```python
from build123d import *

# Parameters (mm, degrees)
SKETCH1_W           = 30
SKETCH1_H           = 30
BOSS_EXTRUDE1_DEPTH = 1.6
SKETCH2_R           = 0.6
CUT_EXTRUDE1_DEPTH  = 1.6
CIRPATTERN1_COUNT   = 2
CIRPATTERN1_ANGLE   = 90
SKETCH4_R           = 0.6
BOSS_EXTRUDE2_DEPTH = 4


with BuildPart() as part:
    # Sketch1 → Boss-Extrude1 (new body)
    with BuildSketch(Plane(origin=(0, 0, 0), x_dir=(1, 0, 0), z_dir=(0, 1, 0))):
        with Locations((15, 15)):
            Rectangle(SKETCH1_W, SKETCH1_H)
    extrude(amount=BOSS_EXTRUDE1_DEPTH)

    # Sketch2 → Cut-Extrude1 (cut)
    with BuildSketch(Plane(origin=(0, 1.6, 0), x_dir=(1, 0, 0), z_dir=(0, 1, 0))):
        with Locations((20.5, 5)):
            Circle(SKETCH2_R)
        with Locations((9.5, 5)):
            Circle(SKETCH2_R)
        with Locations((20.5, 25)):
            Circle(SKETCH2_R)
        with Locations((9.5, 25)):
            Circle(SKETCH2_R)
    cut_extrude1 = extrude(amount=-CUT_EXTRUDE1_DEPTH, mode=Mode.SUBTRACT)

    # CirPattern1: Cut-Extrude1 ×2 about axis
    cirpattern1_axis = Axis((15, 0, -15), (0, 1, 0))
    for i in range(1, CIRPATTERN1_COUNT):
        add(cut_extrude1.rotate(cirpattern1_axis, i * CIRPATTERN1_ANGLE / (CIRPATTERN1_COUNT - 1)), mode=Mode.SUBTRACT)

    # Sketch4 → Boss-Extrude2 (add)
    with BuildSketch(Plane(origin=(0, 1.6, 0), x_dir=(1, 0, 0), z_dir=(0, 1, 0))):
        with Locations((15, 15)):
            Circle(SKETCH4_R)
    extrude(amount=BOSS_EXTRUDE2_DEPTH)


solid = part.part
```
Input: part model. Units: mm. Frame: model coordinates. Round coordinates to 2 decimals unless told otherwise and drop trailing zeros. Loops run counter-clockwise (first coordinate to the right, second up) from the corner with the lowest first, then second, coordinate; pieces in that order, holes last. Notation, with made-up numbers: (4.25, -40) -> (61.25, -40) arc R25 ccw to (61.25, -1) -> close; hole circle Ø8 at (2, 54). An arc over 180 degrees is marked (long way). Use one line per item in the form item = value. Start each with the question number.
Item 1: Section query D-D on y = 2.3. Return the cut outline in (x, z).
Item 2: Contact query for flat-ended pins moving along their axis: pin 1 Ø8 at (x, z) = (4.5, -12) entering from +Y; pin 2 Ø1.4 at (x, z) = (5, -20.5) entering from -Y; pin 3 Ø0.7 at (x, z) = (20.5, -25) entering from +Y. Output: stop coordinate, or through.
Item 3: Section query A-A on z = -25. Return the cut outline in (x, y), then the cut area to 3 significant figures.
Item 4: Mould query, pull axis Z, two halves, no side actions, for faces 1 (the face through (11, 1.6, -15)), 2 (the face through (24.494, 0.811, -20.823)), 3 (the face through (15.572, 3.572, -15.18)). Classes: pulls with the +Z half, pulls with the -Z half, needs draft (parallel to the pull), parting line crosses it, or undercut.
Item 5: Section query C-C on x = 15. Return the cut outline in (y, z).
Item 6: Section query B-B on x = 9.5. Return the cut outline in (y, z).
Item 7: Material intervals for L1, parallel to X at y = 0.6, z = -9.5; L2, parallel to Z at x = 9.5, y = 0.85; L3, parallel to X at y = 1.3, z = -25, sorted ascending. Write a range as from..to.
Ans:
q1.outline = circle Ø1.2 at (15, -15)
q2.pin_1 = 1.6
q2.pin_2 = 0
q2.pin_3 = through
q3.outline = (0, 0) -> (8.9, 0) -> (8.9, 1.6) -> (0, 1.6) -> close; (10.1, 0) -> (19.9, 0) -> (19.9, 1.6) -> (10.1, 1.6) -> close; (21.1, 0) -> (30, 0) -> (30, 1.6) -> (21.1, 1.6) -> close
q3.area = 44.2 mm^2
q4.face_1 = needs draft
q4.face_2 = undercut
q4.face_3 = parting line crosses it
q5.outline = (0, -30) -> (1.6, -30) -> (1.6, -15.6) -> (5.6, -15.6) -> (5.6, -14.4) -> (1.6, -14.4) -> (1.6, 0) -> (0, 0) -> close
q6.outline = (0, -30) -> (1.6, -30) -> (1.6, -25.6) -> (0, -25.6) -> close; (0, -24.4) -> (1.6, -24.4) -> (1.6, -5.6) -> (0, -5.6) -> close; (0, -4.4) -> (1.6, -4.4) -> (1.6, 0) -> (0, 0) -> close
q7.L1 = 0..4.4, 5.6..24.4, 25.6..30
q7.L2 = -30..-25.6, -24.4..-5.6, -4.4..0
q7.L3 = 0..8.9, 10.1..19.9, 21.1..30
